Input: part model. Units: mm. Frame: model coordinates. A direction names the side the tool comes from. Give positions to 0.01 mm unless a question says otherwise; leave off trailing zeros. Loops run counter-clockwise (first coordinate to the right, second up) from the corner with the lowest first, then second, coordinate; pieces in that order, holes last. Notation, with made-up numbers: (21, 53.25) -> (51, 53.25) arc R13 cw to (51, 78.25) -> close; hole circle Ø11 at (51, 22). An arc over 180 degrees is marked (long way). Answer as a JSON object with one key per item and string values.
```python
from build123d import *

# Parameters (mm, degrees)
BOSS_EXTRUDE1_DEPTH = 70
CUT_EXTRUDE1_DEPTH  = 200.200903612
FILLET1_R           = 25


with BuildPart() as part:
    # Sketch1 → Boss-Extrude1 (new body)
    with BuildSketch(Plane.XY):
        with BuildLine():
            Line((-83, 5), (-83, 65))
            ThreePointArc((-83, 65), (-77.142135624, 79.142135624), (-63, 85))
            Line((-63, 85), (63, 85))
            ThreePointArc((63, 85), (77.142135624, 79.142135624), (83, 65))
            Line((83, 65), (83, 5))
            Line((83, 5), (80, 5))
            Line((80, 5), (80, 65))
            ThreePointArc((80, 65), (75.02081528, 77.02081528), (63, 82))
            Line((63, 82), (-63, 82))
            ThreePointArc((-63, 82), (-75.02081528, 77.02081528), (-80, 65))
            Line((-80, 65), (-80, 5))
            Line((-80, 5), (-83, 5))
        make_face()
    extrude(amount=BOSS_EXTRUDE1_DEPTH)

    # Sketch2 → Cut-Extrude1 (cut, through all)
    with BuildSketch(Plane.ZY.offset(83)):
        Polygon((49.016155383, 85), (70, 40), (70, 85), align=None)
        Polygon((10.397928219, 85), (35, 32.240686807), (35, 4.870884332), (0, 4.870884332), (0, 85), align=None)
    extrude(amount=-CUT_EXTRUDE1_DEPTH, mode=Mode.SUBTRACT)

    # Fillet1
    fillet1_edges = [part.edges().sort_by_distance(p)[0] for p in [
        (-81.5, 40, 70),
        (81.5, 40, 70),
        (-81.5, 32.240686807, 35),
        (81.5, 32.240686807, 35),
    ]]
    fillet(fillet1_edges, radius=FILLET1_R)


solid = part.part
```
Q1. Access query for faces 4 (the flat face through (82, 5, 52)), 5 (the cylindrical face through (-74.89, 77.15, 34.74)), 6 (the flat face through (-82, 16, 35)). Directions: +Z, -Z, +X, -X, +Y, -Y. A direction counts if a zero-diameter tool reaches every point of the face in a straight line with its end or side. Return the directions, or none.
Evaluation:
{"face 4": "+Z, -Z, +X, -X, -Y", "face 5": "+Z, -Z, -Y", "face 6": "-Z, +X, -X, -Y"}
Q2. Section C-C, the plane z = 63. Return the cut outline in (x, y), then the cut area to 3 significant figures.
Evaluation:
{"outline": "(-83, 5) -> (-80, 5) -> (-80, 55.01) -> (-83, 55.01) -> close; (80, 5) -> (83, 5) -> (83, 55.01) -> (80, 55.01) -> close", "area": "300 mm2"}
Q3. Section B-B, the plane z = 46. Return the cut outline in (x, y).
Evaluation:
{"outline": "(-83, 5) -> (-80, 5) -> (-80, 65) arc R17 cw to (-63, 82) -> (63, 82) arc R17 cw to (80, 65) -> (80, 5) -> (83, 5) -> (83, 65) arc R20 ccw to (63, 85) -> (-63, 85) arc R20 ccw to (-83, 65) -> close"}
Q4. Ray query, line 1 along X through (y, z) = (47, 42); line 2 along Y through (x, z) = (27, 47.5); line 3 along X through (y, z) = (67, 40). Return the intervals inside material, ascending.
Evaluation:
{"line 1": "x = -83 to -80, 80 to 83", "line 2": "y = 82 to 85", "line 3": "x = -82.9 to -79.88, 79.88 to 82.9"}
Q5. Pin query (flat end, axial travel): pin 1 (10 mm diameter, centred on y = 76, z = 40.5, fed in from -X); pin 2 (3.5 mm diameter, centred on x = 81, y = 16, fed in from -Z); pin 3 (11.5 mm diameter, centred on x = 3.5, z = 31.5, fed in from -Y). Return the tip coordinate at first contact, or that it passes through.
Evaluation:
{"pin 1": "stops at x = -82.08", "pin 2": "stops at z = 35", "pin 3": "stops at y = 82"}
Q6. Draft query along X for faces 1 (the cylindrical face through (81.52, 32.18, 34.39)), 2 (the flat face through (-83, 35, 50)), 3 (the flat face through (80, 35, 50)). Return one class per face: +X half, -X half, draft (parallel to the pull), parting line (faces both ways), or undercut.
Evaluation:
{"face 1": "draft", "face 2": "-X half", "face 3": "undercut"}
Q7. Section D-D, the plane x = -32. Return the cut outline in (y, z), then the cut area to 3 significant figures.
Evaluation:
{"outline": "(82, 11.8) -> (85, 10.4) -> (85, 49.02) -> (82, 50.42) -> close", "area": "116 mm2"}
Q8. Section A-A, the plane y = 19. Return the cut outline in (x, z), then the cut area to 3 significant figures.
Evaluation:
{"outline": "(-83, 35) -> (-80, 35) -> (-80, 70) -> (-83, 70) -> close; (80, 35) -> (83, 35) -> (83, 70) -> (80, 70) -> close", "area": "210 mm2"}
